from build123d import *

# Parameters (mm, degrees)
F0_R     = 1.8
F1_DEPTH = 4
F2_DEPTH = 6
F4_SIZE  = 1
F3_R     = 1.25
F5_DEPTH = 40


with BuildPart() as f1:
    # F0 (on Top) → F1 (new body)
    with BuildSketch(Plane.XY):
        Polygon((4, 22), (-4, 22), (-4, -10), (0, -10), (4, -10), align=None)
        Circle(F0_R, mode=Mode.SUBTRACT)
    extrude(amount=F1_DEPTH)

    # F0 (on Top) → F2 (join)
    with BuildSketch(Plane.XY):
        Polygon((8, 26), (0, 26), (-8, 26), (-8, 22), (-4, 22), (4, 22), (8, 22), align=None)
    extrude(amount=F2_DEPTH)

    # F4
    f4_edges = [f1.edges().sort_by_distance(p)[0] for p in [
        (0, 22, 6),
        (-4, 6, 4),
        (4, 6, 4),
    ]]
    chamfer(f4_edges, length=F4_SIZE)

    # F3 (on face) → F5 (cut)
    with BuildSketch(Plane(origin=(0, 26, 0), x_dir=(-1, 0, 0), z_dir=(0, 1, 0))):
        with Locations((-5, 3)):
            Circle(F3_R)
        with Locations((5, 3)):
            Circle(F3_R)
    extrude(amount=-F5_DEPTH, mode=Mode.SUBTRACT)


solid = f1.part
Can you work these out from the model? Positions are in its coordinate system, mm. A direction names the side the tool comes from. Give positions to 0.01 mm unless a question says otherwise; leave off trailing zeros. Write each loop counter-clockwise with the first axis right and the second up, starting at its lowest first coordinate (ties: lowest second). Pieces come first, ordered by that corner, then holes. Notation, with made-up numbers: M 80,18.25 L 132,18.25 A10 ccw 132,37.25 Z; hole C 19.5,-3 d2. An arc over 180 degrees is marked long. Answer in a Markdown table with one row per item. Add a question column.
Item 1: Imagine slicing it at B-B, the plane x = 5. Write out the boundary of the cut face in (y, z), plus the area to 3 significant figures.
Item 2: We'd pull the mould along X, two halves only. Please class faces 1 (the flat face through (8, 24, 3)), 2 (the cylindrical face through (1.717, 0.541, 1.972)), 3 (the flat face through (-0.1, 22.5, 5.5)), 4 (the flat face through (-8, 24, 3)): released by +X, released by -X, zero draft, split by the parting line, or undercut.
Item 3: On a 3-axis mill with a long thin cutter (end or side, diameter ignored), from which of +Z, -Z, +X, -X, +Y, -Y can I reach the whole of each face in a straight line? I mean faces 5 (the flat face through (4, 6, 1)), 6 (the flat face through (-4, 6, 1)), 7 (the flat face through (-0.1, 22, 4.7)). Say none if no direction works.
Item 4: Imagine slicing it at A-A, the plane y = 0. Write out the boundary of the cut face in (x, z), plus the area to 3 significant figures.
Item 5: Imagine slicing it at D-D, the plane x = 0. Write out the boundary of the cut face in (y, z), plus the area to 3 significant figures.
Item 6: Imagine slicing it at C-C, the plane z = 0.5. Write out the boundary of the cut face in (x, y).
Item 7: Please list where these lines run through material, in increasing order: L1, parallel to Y at x = 0, z = 1.9; L2, parallel to Y at x = -4.5, z = 1; L3, parallel to Z at x = 3, y = -2.5.
Item 8: For pin 1 Ø8 at (x, y) = (3.5, 5) entering from +Z; pin 2 Ø1.5 at (x, z) = (5, 3) entering from -Y; pin 3 Ø1.8 at (y, z) = (12, 1) entering from +X; pin 4 Ø0.7 at (y, z) = (2, 1) entering from -X, each with a flat end and sliding along its axis, tell me the tip position at first contact or that it passes through.
Evaluation:
| question | item | result |
|---|---|---|
| 1 | outline | M 22,0 L 26,0 L 26,1.75 L 22,1.75 Z; M 22,4.25 L 26,4.25 L 26,6 L 23,6 L 22,5 Z |
| 1 | area | 13.5 mm² |
| 2 | face 1 | released by +X |
| 2 | face 2 | undercut |
| 2 | face 3 | zero draft |
| 2 | face 4 | released by -X |
| 3 | face 5 | +Z, -Z, +X, -Y |
| 3 | face 6 | +Z, -Z, -X, -Y |
| 3 | face 7 | +Z, -Y |
| 4 | outline | M -4,0 L -1.8,0 L -1.8,4 L -3,4 L -3.77,3.23 A1.25 cw -4,2.25 Z; M 1.8,0 L 4,0 L 4,2.25 A1.25 cw 3.77,3.23 L 3,4 L 1.8,4 Z |
| 4 | area | 16.3 mm² |
| 5 | outline | M -10,0 L -1.8,0 L -1.8,4 L -10,4 Z; M 1.8,0 L 26,0 L 26,6 L 23,6 L 22,5 L 22,4 L 1.8,4 Z |
| 5 | area | 137 mm² |
| 6 | outline | M -8,22 L -4,22 L -4,-10 L 4,-10 L 4,22 L 8,22 L 8,26 L -8,26 Z; hole C 0,0 d3.6 |
| 7 | L1 | y = -10 to -1.8, 1.8 to 26 |
| 7 | L2 | y = 22 to 26 |
| 7 | L3 | z = 0 to 4 |
| 8 | pin 1 | stops at z = 4 |
| 8 | pin 2 | passes through |
| 8 | pin 3 | stops at x = 4 |
| 8 | pin 4 | stops at x = -4 |
